Build history of the part. All positions in model axes, mm. A direction names the side the tool comes from. Give positions to 0.01 mm unless a question says otherwise; leave off trailing zeros. Loops run counter-clockwise (first coordinate to the right, second up) from the corner with the lowest first, then second, coordinate; pieces in that order, holes last. Notation, with made-up numbers: M 17,-11.75 L 47,-11.75 A23 ccw 47,26.25 Z; hole C 60.5,42 d2. An arc over 180 degrees is marked long. Put each result on its own line as item: value.
```python
from build123d import *

# Parameters (mm, degrees)
SKETCH1_R           = 4
SKETCH1_R_2         = 1.5
SKETCH1_R_3         = 2
BOSS_EXTRUDE1_DEPTH = 2.5
SKETCH2_R           = 2.1
BOSS_EXTRUDE2_DEPTH = 9.5
SKETCH4_R           = 1.5
CUT_EXTRUDE1_DEPTH  = 5


with BuildPart() as part:
    # Sketch1 → Boss-Extrude1 (new body)
    with BuildSketch(Plane.XY):
        with BuildLine():
            Line((-24, 5.07179677), (-24, 21.07179677))
            Line((-24, 21.07179677), (-4, 33.07179677))
            Line((-4, 33.07179677), (4, 33.07179677))
            Line((4, 33.07179677), (24, 21.07179677))
            Line((24, 21.07179677), (24, 5.07179677))
            Line((24, 5.07179677), (8, -6.92820323))
            Line((8, -6.92820323), (8, -34.92820323))
            ThreePointArc((8, -34.92820323), (7.414213562, -36.342416793), (6, -36.92820323))
            Line((6, -36.92820323), (-6, -36.92820323))
            ThreePointArc((-6, -36.92820323), (-7.414213562, -36.342416793), (-8, -34.92820323))
            Line((-8, -34.92820323), (-8, -6.92820323))
            Line((-8, -6.92820323), (-24, 5.07179677))
        make_face()
        with Locations((-12, 12.07179677)):
            Circle(SKETCH1_R, mode=Mode.SUBTRACT)
        with Locations((-5, 12.07179677)):
            Circle(SKETCH1_R_2, mode=Mode.SUBTRACT)
        with Locations((5, 12.07179677)):
            Circle(SKETCH1_R_2, mode=Mode.SUBTRACT)
        with Locations((0, 27.07179677)):
            Circle(SKETCH1_R_2, mode=Mode.SUBTRACT)
        with Locations((20, 17.07179677)):
            Circle(SKETCH1_R_2, mode=Mode.SUBTRACT)
        with Locations((20, 9.07179677)):
            Circle(SKETCH1_R_2, mode=Mode.SUBTRACT)
        with Locations((-20, 17.07179677)):
            Circle(SKETCH1_R_2, mode=Mode.SUBTRACT)
        with Locations((-20, 9.07179677)):
            Circle(SKETCH1_R_2, mode=Mode.SUBTRACT)
        with Locations((13, 12.07179677)):
            Circle(SKETCH1_R_3, mode=Mode.SUBTRACT)
        with BuildLine():
            Line((4, -30.92820323), (-4, -30.92820323))
            Line((-4, -30.92820323), (-4, -6.92820323))
            ThreePointArc((-4, -6.92820323), (0, 8), (4, -6.92820323))
            Line((4, -6.92820323), (4, -30.92820323))
        make_face(mode=Mode.SUBTRACT)
        with BuildLine():
            Line((-5, 23.07179677), (5, 23.07179677))
            ThreePointArc((5, 23.07179677), (6.414213562, 22.486010332), (7, 21.07179677))
            Line((7, 21.07179677), (7, 18.07179677))
            ThreePointArc((7, 18.07179677), (6.414213562, 16.657583207), (5, 16.07179677))
            Line((5, 16.07179677), (-5, 16.07179677))
            ThreePointArc((-5, 16.07179677), (-6.414213562, 16.657583207), (-7, 18.07179677))
            Line((-7, 18.07179677), (-7, 21.07179677))
            ThreePointArc((-7, 21.07179677), (-6.414213562, 22.486010332), (-5, 23.07179677))
        make_face(mode=Mode.SUBTRACT)
    extrude(amount=BOSS_EXTRUDE1_DEPTH)

    # Sketch2 → Boss-Extrude2 (add)
    with BuildSketch(Plane(origin=(0, 0, 0), x_dir=(-1, 0, 0), z_dir=(0, 0, -1))):
        with Locations(Location((-5, -33.42820323, 0), (0, 0, 180))):
            Circle(SKETCH2_R)
        with Locations(Location((5, -33.42820323, 0), (0, 0, 180))):
            Circle(SKETCH2_R)
    extrude(amount=BOSS_EXTRUDE2_DEPTH)

    # Sketch4 → Cut-Extrude1 (cut)
    with BuildSketch(Plane(origin=(0, 0, -9.5), x_dir=(-1, 0, 0), z_dir=(0, 0, -1))):
        with Locations((-5, -33.42820323)):
            Circle(SKETCH4_R)
        with Locations((5, -33.42820323)):
            Circle(SKETCH4_R)
    extrude(amount=-CUT_EXTRUDE1_DEPTH, mode=Mode.SUBTRACT)


solid = part.part
```
Q1. Drop flat-ended pins along their axis: pin 1 Ø3.5 at (x, y) = (-5.5, -34) entering from -Z; pin 2 Ø2.5 at (x, y) = (-5, -33.43) entering from -Z; pin 3 Ø3.5 at (x, y) = (-5, 12.07) entering from -Z; pin 4 Ø3 at (y, z) = (-17, 1) entering from -X. Give the stop position or say it passes through.
Here are the results:
pin 1: z = -9.5
pin 2: z = -4.5
pin 3: z = 0
pin 4: x = -8
Q2. Tool access for faces 1 (the flat face through (-5, -33, -4.5)), 2 (the flat face through (-7, 20, 1)), 3 (the flat face through (8, -21, 1)), 4 (the flat face through (6.4, -32.5, -9.5)), 5 (the flat face through (-8, -21, 1)): list every direction of +Z, -Z, +X, -X, +Y, -Y with a clear straight run to the whole face (end or side of a thin tool).
Here are the results:
face 1: -Z
face 2: +Z, -Z
face 3: +Z, -Z, +X, -Y
face 4: -Z, +X, -X, +Y, -Y
face 5: +Z, -Z, -X, -Y
Q3. Slice it at C-C (z = 1.5). State how many separate pieces and enclosed holes the cut face has, and give its area (3 significant figures).
Here are the results:
separate pieces: 1
enclosed holes: 11
area: 1,370 mm²
Q4. Slice it at B-B (x = 0). List the corners of the cut face in (y, z).
Here are the results:
outline: M -36.93,0 L -30.93,0 L -30.93,2.5 L -36.93,2.5 Z; M 8,0 L 16.07,0 L 16.07,2.5 L 8,2.5 Z; M 23.07,0 L 25.57,0 L 25.57,2.5 L 23.07,2.5 Z; M 28.57,0 L 33.07,0 L 33.07,2.5 L 28.57,2.5 Z
Q5. Slice it at A-A (y = -10.5). List the corners of the cut face in (x, z), and give its area (3 significant figures).
Here are the results:
outline: M -8,0 L -4,0 L -4,2.5 L -8,2.5 Z; M 4,0 L 8,0 L 8,2.5 L 4,2.5 Z
area: 20.0 mm²
Q6. Slice it at D-D (x = 13). List the corners of the cut face in (y, z).
Here are the results:
outline: M -3.18,0 L 10.07,0 L 10.07,2.5 L -3.18,2.5 Z; M 14.07,0 L 27.67,0 L 27.67,2.5 L 14.07,2.5 Z
Q7. Mould opens along Y. For faces 6 (the cylindrical face through (18.5, 17.1, 1.2)), 7 (the flat face through (24, 13, 1)), 8 (the flat face through (0, 33.072, 1)), 9 (the flat face through (5, -33, -4.5)) say: pulls with the +Y half, pulls with the -Y half, needs draft (parallel to the pull), parting line crosses it, or undercut.
Here are the results:
face 6: undercut
face 7: needs draft
face 8: pulls with the +Y half
face 9: undercut
Q8. Probe line 1 (Y direction, x = 5, z = 1.75) (3 decimals); line 2 (Z direction, x = -4, y = 7); line 3 (X direction, y = -11, z = 1). List the from-to ranges inside material, lowest first. Write a range as from..to.
Here are the results:
line 1: -36.928..-6.245, 6.245..10.572, 13.572..16.072, 23.072..32.472
line 2: 0..2.5
line 3: -8..-4, 4..8
